```python
from build123d import *

# Parameters (mm, degrees)
SKETCH1_W               = 120
SKETCH1_H               = 133
BOSS_EXTRUDE1_DEPTH     = 3
SKETCH2_W               = 120
SKETCH2_H               = 5
BOSS_EXTRUDE2_DEPTH     = 8
SKETCH3_W               = 22
SKETCH3_H               = 10
CUT_EXTRUDE1_DEPTH      = 1
CUT_EXTRUDE1_DEPTH_BACK = 12
SKETCH4_W               = 120
SKETCH4_H               = 5
BOSS_EXTRUDE3_DEPTH     = 11
SKETCH5_W               = 80
SKETCH5_H               = 3
BOSS_EXTRUDE4_DEPTH     = 80
SKETCH6_R               = 1
SKETCH6_R_2             = 5.5
CUT_EXTRUDE2_DEPTH      = 80


with BuildPart() as part:
    # Sketch1 → Boss-Extrude1 (new body)
    with BuildSketch(Plane(origin=(0, 0, 0), x_dir=(1, 0, 0), z_dir=(0, 1, 0))):
        Rectangle(SKETCH1_W, SKETCH1_H)
    extrude(amount=BOSS_EXTRUDE1_DEPTH)

    # Sketch2 → Boss-Extrude2 (add)
    with BuildSketch(Plane(origin=(0, 3, 0), x_dir=(1, 0, 0), z_dir=(0, 1, 0))):
        with Locations((0, -64)):
            Rectangle(SKETCH2_W, SKETCH2_H)
    extrude(amount=BOSS_EXTRUDE2_DEPTH)

    # Sketch3 → Cut-Extrude1 (cut, two sides)
    with BuildSketch(Plane(origin=(0, 11, 0), x_dir=(1, 0, 0), z_dir=(0, 1, 0))) as cut_extrude1_sk:
        with Locations((0, -61.5)):
            Rectangle(SKETCH3_W, SKETCH3_H)
    extrude(amount=CUT_EXTRUDE1_DEPTH, mode=Mode.SUBTRACT)
    extrude(cut_extrude1_sk.sketch, amount=-CUT_EXTRUDE1_DEPTH_BACK, mode=Mode.SUBTRACT)

    # Sketch4 → Boss-Extrude3 (add)
    with BuildSketch(Plane(origin=(0, 0, 0), x_dir=(1, 0, 0), z_dir=(0, 1, 0))):
        with Locations((0, 69)):
            Rectangle(SKETCH4_W, SKETCH4_H)
    extrude(amount=BOSS_EXTRUDE3_DEPTH)

    # Sketch5 → Boss-Extrude4 (add)
    with BuildSketch(Plane(origin=(0, 0, 0), x_dir=(0, 0, -1), z_dir=(1, 0, 0))):
        with Locations((11.5, 1.5)):
            Rectangle(SKETCH5_W, SKETCH5_H)
    boss_extrude4 = extrude(amount=BOSS_EXTRUDE4_DEPTH)

    # Sketch6 → Cut-Extrude2 (cut)
    with BuildSketch(Plane(origin=(0, 3, 0), x_dir=(1, 0, 0), z_dir=(0, 1, 0))):
        with Locations((70, 11.5)):
            Circle(SKETCH6_R)
        with Locations((70, 31.5)):
            Circle(SKETCH6_R_2)
        with Locations((70, -8.5)):
            Circle(SKETCH6_R_2)
    cut_extrude2 = extrude(amount=-CUT_EXTRUDE2_DEPTH, mode=Mode.SUBTRACT)

    # Mirror1: Boss-Extrude4, Cut-Extrude2 across plane
    add(boss_extrude4.mirror(Plane(origin=(0, 0, 0), x_dir=(0, 0, 1), z_dir=(1, 0, 0))))
    add(cut_extrude2.mirror(Plane(origin=(0, 0, 0), x_dir=(0, 0, 1), z_dir=(1, 0, 0))), mode=Mode.SUBTRACT)


solid = part.part
```
Can you work these out from the model? Positions are in its coordinate system, mm. A direction names the side the tool comes from. Give positions to 0.01 mm unless a question says otherwise; leave off trailing zeros. Order: outer loops, then holes, each group sorted by start corner. A loop starts at its lowest first (then second) coordinate and runs counter-clockwise, first axis right, second up. Notation, with made-up numbers: M -32,87 L -6,87 A28 cw -6,105 Z; hole C 56.25,44 d8. An arc over 180 degrees is marked long. One line per item, written item: value.
1) I want a section at C-C, the plane x = -47. List the corners of the cut face in (y, z) for me.
Answer sheet:
outline: M 0,-71.5 L 11,-71.5 L 11,-66.5 L 3,-66.5 L 3,61.5 L 11,61.5 L 11,66.5 L 0,66.5 Z
2) We'd pull the mould along Z, two halves only. Please class faces 6 (the face through (-1, 5, -71.5)), 7 (the face through (-64.505, 1.521, 8.258)), 8 (the face through (60, 2, 52)): released by +Z, released by -Z, zero draft, split by the parting line, or undercut.
Answer sheet:
face 6: released by -Z
face 7: undercut
face 8: zero draft
3) Please list where these lines run through material, in increasing order: line 1 along Z through (x, y) = (70, 1.8); line 2 along X through (y, z) = (2.35, -11.5); line 3 along Z through (x, y) = (34.5, 6.5).
Answer sheet:
line 1: z = -51.5 to -37, -26 to -12.5, -10.5 to 3, 14 to 28.5
line 2: x = -80 to -71, -69 to 69, 71 to 80
line 3: z = -71.5 to -66.5, 61.5 to 66.5
4) I want a section at A-A, the plane z = -31.5. List the corners of the cut face in (x, y) for me, plus the area to 3 significant figures.
Answer sheet:
outline: M -80,0 L -75.5,0 L -75.5,3 L -80,3 Z; M -64.5,0 L 64.5,0 L 64.5,3 L -64.5,3 Z; M 75.5,0 L 80,0 L 80,3 L 75.5,3 Z
area: 414 mm^2
5) I want a section at B-B, the plane y = 6.25. List the corners of the cut face in (x, z) for me.
Answer sheet:
outline: M -60,-71.5 L 60,-71.5 L 60,-66.5 L -60,-66.5 Z; M -60,61.5 L -11,61.5 L -11,66.5 L -60,66.5 Z; M 11,61.5 L 60,61.5 L 60,66.5 L 11,66.5 Z
6) For P1, Ø2.5, axis at x = -70, z = -11.5, coming from the +Y side; P2, Ø3.5, axis at x = 71.5, y = 2, coming from the -Z side; P3, Ø5.5, axis at y = 3.5, z = 46.5, coming from the +X side; P4, Ø6.5, axis at x = 70, z = -31.5, coming from the +Y side, each with a flat end and sliding along its axis, tell me the tip position at first contact or that it passes through.
Answer sheet:
P1: stops at y = 3
P2: stops at z = -51.5
P3: stops at x = 60
P4: passes through
7) On a 3-axis mill with a long thin cutter (end or side, diameter ignored), from which of +Z, -Z, +X, -X, +Y, -Y can I reach the whole of each face in a straight line? I mean faces 1 (the face through (-60, 2, 52)), 2 (the face through (-60, 2, -64)), 3 (the face through (-36, 7, 61.5)), 4 (the face through (11, 4, 63)), 5 (the face through (-36, 5, 66.5)). Say none if no direction works.
Answer sheet:
face 1: +Z, -X, +Y, -Y
face 2: -Z, -X, +Y, -Y
face 3: +X, -X, +Y
face 4: +Z, +Y, -Y
face 5: +Z, +X, -X, +Y, -Y
